from build123d import *

# Parameters (mm, degrees)
RESSALTO_EXTRUS_O1_DEPTH = 3
RESSALTO_EXTRUS_O2_DEPTH = 5
FILETE1_R                = 5


with BuildPart() as part:
    # Esboço1 → Ressalto-extrusão1 (new body)
    with BuildSketch(Plane.XY):
        with BuildLine():
            Line((-40, 0), (-40, 200))
            Line((-40, 200), (40, 200))
            Line((40, 200), (40, 0))
            ThreePointArc((40, 0), (0, -40), (-40, 0))
        make_face()
    extrude(amount=RESSALTO_EXTRUS_O1_DEPTH)

    # Esboço2 → Ressalto-extrusão2 (add)
    with BuildSketch(Plane.XY.offset(3)):
        with BuildLine():
            Line((-34.9, 0), (-34.9, 194.9))
            Line((-34.9, 194.9), (34.9, 194.9))
            Line((34.9, 194.9), (34.9, 0))
            ThreePointArc((34.9, 0), (0, -34.9), (-34.9, 0))
        make_face()
        with BuildLine():
            Line((32, 0), (32, 191.9))
            Line((32, 191.9), (-32, 191.9))
            Line((-32, 191.9), (-32, 0))
            ThreePointArc((-32, 0), (0, -32), (32, 0))
        make_face(mode=Mode.SUBTRACT)
    extrude(amount=RESSALTO_EXTRUS_O2_DEPTH)

    # Filete1
    # the kernel refuses this fillet: 5 mm, written as the material it takes off along each edge
    with BuildSketch(Plane(origin=(40, 211.456439237, 0), x_dir=(-1, 0, 0), z_dir=(0, -1, 0))) as filete1_piece_1:
        with BuildLine():
            CenterArc((4.582575695, -5), FILETE1_R, 90, 66.421821522)
            Line((0, -3), (-0.091651514, -2.96))
            ThreePointArc((-0.091651514, -2.96), (-0.1, -1.5), (-0.1, 0))
            Line((-0.1, 0), (0, 0.1))
            Line((0, 0.1), (4.582575695, 0.1))
            Line((4.582575695, 0.1), (4.582575695, 0))
        make_face()
    extrude(amount=211.456439237, mode=Mode.SUBTRACT)
    with BuildSketch(Plane(origin=(0, 0, 0), x_dir=(1, 0, 0), z_dir=(0, 1, 0))) as filete1_piece_2:
        with BuildLine():
            CenterArc((35.417424305, -5), FILETE1_R, 23.578178478, 66.421821522)
            Line((35.417424305, 0), (35.417424305, 0.1))
            Line((35.417424305, 0.1), (40, 0.1))
            Line((40, 0.1), (40.1, 0))
            ThreePointArc((40.1, 0), (40.1, -1.5), (40.091651514, -2.96))
            Line((40.091651514, -2.96), (40, -3))
        make_face()
    revolve(axis=Axis((0, 0, 0), (0, 0, -1)), revolution_arc=180, mode=Mode.SUBTRACT)
    with BuildSketch(Plane(origin=(-40, 0, 0), x_dir=(0, 0, 1), z_dir=(0, 1, 0))) as filete1_piece_3:
        with BuildLine():
            CenterArc((5, 4.582575695), FILETE1_R, 180, 66.421821522)
            Line((0, 4.582575695), (-0.1, 4.582575695))
            Line((-0.1, 4.582575695), (-0.1, 0))
            Line((-0.1, 0), (0, -0.1))
            ThreePointArc((0, -0.1), (1.5, -0.1), (2.96, -0.091651514))
            Line((2.96, -0.091651514), (3, 0))
        make_face()
    extrude(amount=211.456439237, mode=Mode.SUBTRACT)


solid = part.part
Model file for the job. Use its own axes, mm. A direction names the side the tool comes from. Round coordinates to 2 decimals unless told otherwise and drop trailing zeros. Loops run counter-clockwise (first coordinate to the right, second up) from the corner with the lowest first, then second, coordinate; pieces in that order, holes last. Notation, with made-up numbers: (29.5, 42) - (68.5, 42) arc R7 cw to (68.5, 52) - close; hole circle Ø4 at (79, 12). An arc over 180 degrees is marked (long way). Write each question's results on one line, items separated by ' | '.
(1) Mould opens along X. For faces 1 (the flat face through (34.9, 99, 5)), 2 (the flat face through (-32, 97, 5)), 3 (the cylindrical face through (-38.122, 98.6, 0.795)), 4 (the flat face through (32, 95, 5)) say: released by +X, released by -X, zero draft, split by the parting line, or undercut.
Answer below:
face 1: released by +X | face 2: undercut | face 3: released by -X | face 4: undercut
(2) 3-axis set-ups, long thin cutter, end or side, ignore diameter. For faces 5 (the cylindrical face through (-0.704, -31.992, 5.465)), 6 (the cylindrical face through (0.77, -34.89, 5.46)), 7 (the flat face through (-34.9, 96, 5)): which of +Z, -Z, +X, -X, +Y, -Y reach the whole face in a straight line?
Answer below:
face 5: +Z | face 6: +Z, -Y | face 7: +Z, -X, +Y, -Y
(3) Pin check, flat tips, straight feed: pin 1 (2 mm diameter, centred on x = 17, y = 37, fed in from +Z); pin 2 (1.5 mm diameter, centred on y = 126.5, z = 4.5, fed in from +X); pin 3 (2.5 mm diameter, centred on y = 108.5, z = 5.5, fed in from -X). Stop position of each tip, or through.
Answer below:
pin 1: stops at z = 3 | pin 2: stops at x = 34.9 | pin 3: stops at x = -34.9
(4) Wall check: L1, parallel to X at y = 107.5, z = 3.5; L2, parallel to Z at x = 4.5, y = 8; L3, parallel to Y at x = 11, z = 5.75. Give the ranges that are in metal, low to high.
Answer below:
L1: x = -34.9 to -32, 32 to 34.9 | L2: z = 0 to 3 | L3: y = -33.12 to -30.05, 191.9 to 194.9
(5) Saw through at B-B, the plane z = 6.75. List the corners of the cut face in (x, y).
Answer below:
outline: (-34.9, 0) arc R34.9 ccw to (34.9, 0) - (34.9, 194.9) - (-34.9, 194.9) - close; hole (-32, 0) arc R32 ccw to (32, 0) - (32, 191.9) - (-32, 191.9) - close
(6) Saw through at C-C, the plane y = 54.5. List the corners of the cut face in (x, z).
Answer below:
outline: (-40, 3) arc R5 ccw to (-35.42, 0) - (35.42, 0) arc R5 ccw to (40, 3) - (34.9, 3) - (34.9, 8) - (32, 8) - (32, 3) - (-32, 3) - (-32, 8) - (-34.9, 8) - (-34.9, 3) - close
(7) Saw through at A-A, the plane x = 0. List the corners of the cut face in (y, z).
Answer below:
outline: (-40, 3) arc R5 ccw to (-35.42, 0) - (200, 0) - (200, 3) - (194.9, 3) - (194.9, 8) - (191.9, 8) - (191.9, 3) - (-32, 3) - (-32, 8) - (-34.9, 8) - (-34.9, 3) - close
